Design review of the part built by this model. Coordinates are the model's own, in mm. Give positions to 0.01 mm unless a question says otherwise; leave off trailing zeros. Order: outer loops, then holes, each group sorted by start corner. A loop starts at its lowest first (then second) coordinate and runs counter-clockwise, first axis right, second up. Notation, with made-up numbers: M 49,-31 L 104,-31 A32 ccw 104,3 Z; hole C 33,75 d2. An arc over 180 degrees is marked long. Answer as a JSON object with one key per item and string values.
from build123d import *

# Parameters (mm, degrees)
PAD008_DEPTH          = 5
SKETCH022_W           = 88.2
SKETCH022_H           = 88.2
SKETCH022_R           = 2.5
PAD009_DEPTH          = 1.8
CHAMFER004_SIZE       = 1.2
PAD010_DEPTH          = 44.1
POCKET006_DEPTH       = 256.838707
POLARPATTERN002_COUNT = 8
CHAMFER005_SIZE       = 1.5
FILLET003_R           = 1.19


with BuildPart() as part:
    # Sketch021 → Pad008 (new body)
    with BuildSketch(Plane.XY.offset(-0.2)):
        Polygon((-42.9, 42.9), (-42.9, -42.9), (42.9, -42.9), (42.9, 42.9), (42.9, 44.1), (44.1, 44.1), (44.1, -44.1), (-44.1, -44.1), (-44.1, 44.1), (-42.9, 44.1), align=None)
    extrude(amount=-PAD008_DEPTH)

    # Sketch022 → Pad009 (join)
    with BuildSketch(Plane.XY.offset(-5.2)):
        Rectangle(SKETCH022_W, SKETCH022_H)
        with Locations((-35.7, 35.7)):
            Circle(SKETCH022_R, mode=Mode.SUBTRACT)
        with Locations((35.7, 35.7)):
            Circle(SKETCH022_R, mode=Mode.SUBTRACT)
        with Locations((35.7, -35.7)):
            Circle(SKETCH022_R, mode=Mode.SUBTRACT)
        with Locations((-35.7, -35.7)):
            Circle(SKETCH022_R, mode=Mode.SUBTRACT)
    extrude(amount=-PAD009_DEPTH)

    # Chamfer004
    chamfer004_edges = [part.edges().sort_by_distance(p)[0] for p in [
        (-38.2, 35.7, -7),
        (-38.2, -35.7, -7),
        (33.2, -35.7, -7),
        (33.2, 35.7, -7),
    ]]
    chamfer(chamfer004_edges, length=CHAMFER004_SIZE)

    # Sketch023 → Pad010 (join, symmetric)
    with BuildSketch(Plane.XZ):
        Polygon((42.9, -0.2), (42.9, -2.6), (41.7, -1.4), align=None)
        Polygon((-42.9, -0.2), (-42.9, -2.6), (-41.7, -1.4), align=None)
    extrude(amount=PAD010_DEPTH, both=True)

    # Sketch024 → Pocket006 (cut, through all)
    with BuildSketch(Plane.XY):
        with BuildLine():
            ThreePointArc((27.005677, 28.137047), (14.924654, 36.031302), (0.8, 38.991794))
            Line((0.8, 38.991794), (0.8, 27.785223))
            ThreePointArc((19.081434, 20.212805), (10.637351, 25.680837), (0.8, 27.785223))
            Line((19.081434, 20.212805), (27.005677, 28.137047))
        make_face()
        with BuildLine():
            ThreePointArc((17.950063, 19.081434), (10.025326, 24.203279), (0.8, 26.185223))
            Line((0.8, 14.978651), (0.8, 26.185223))
            ThreePointArc((10.025821, 11.157191), (5.740251, 13.858193), (0.8, 14.978651))
            Line((10.025821, 11.157191), (17.950063, 19.081434))
        make_face()
    pocket006 = extrude(amount=-POCKET006_DEPTH, mode=Mode.SUBTRACT)

    # PolarPattern002: Pocket006 ×8 about axis
    polarpattern002_axis = Axis((0, 0, 0), (0, 0, 1))
    for i in range(1, POLARPATTERN002_COUNT):
        add(pocket006.rotate(polarpattern002_axis, i * 360 / POLARPATTERN002_COUNT), mode=Mode.SUBTRACT)

    # Chamfer005
    chamfer005_edges = [part.edges().sort_by_distance(p)[0] for p in [
        (-44.1, 0, -7),
        (0, -44.1, -7),
        (44.1, 0, -7),
        (0, 44.1, -7),
    ]]
    chamfer(chamfer005_edges, length=CHAMFER005_SIZE)

    # Fillet003
    fillet003_edges = [part.edges().sort_by_distance(p)[0] for p in [
        (-44.1, 44.1, -2.85),
        (-44.1, -44.1, -2.85),
        (44.1, 44.1, -2.85),
        (44.1, -44.1, -2.85),
    ]]
    fillet(fillet003_edges, radius=FILLET003_R)


solid = part.part
(1) We need section C-C (x = -35.7). Write out the cut boundary in (y, z).
Checked values:
{"outline": "M -44.1,-5.5 L -42.6,-7 L -39.4,-7 L -38.2,-5.8 L -38.2,-5.2 L -42.9,-5.2 L -42.9,-0.2 L -44.1,-0.2 Z; M -33.2,-5.8 L -32,-7 L -15.7,-7 L -15.7,-5.2 L -33.2,-5.2 Z; M -0.8,-7 L 0.8,-7 L 0.8,-5.2 L -0.8,-5.2 Z; M 15.7,-7 L 32,-7 L 33.2,-5.8 L 33.2,-5.2 L 15.7,-5.2 Z; M 38.2,-5.8 L 39.4,-7 L 42.6,-7 L 44.1,-5.5 L 44.1,-5.2 L 38.2,-5.2 Z"}
(2) Draft analysis for pull direction X (two halves, no side actions). For faces 1 (the flat face through (-1, -44.1, -3)), 2 (the cylindrical face through (-5.81, -13.83, -6.09)), 3 (the cylindrical face through (33.2, 35.8, -5.5)), state which applies: +X half, -X half, draft (parallel to the pull), parting line (faces both ways), or undercut.
Checked values:
{"face 1": "draft", "face 2": "undercut", "face 3": "undercut"}
(3) We need section A-A (x = 12.5). Count the separate pieces of the cut face and the enclosed holes in it, plus the area to 3 significant figures.
Checked values:
{"separate pieces": "7", "enclosed holes": "0", "area": "74.0 mm^2"}
(4) To check wall thickness, follow L1, parallel to X at y = 23.5, z = -4.25; L2, parallel to X at y = -35.5, z = -5.75; L3, parallel to Y at x = -33.5, z = -6.5. State the ranges of each line that lie inside material, in increasing order. Write a range as from..to.
Checked values:
{"L1": "x = -44.1..-42.9, 42.9..44.1", "L2": "x = -43.85..-38.19, -33.21..-16.15, -0.8..0.8, 16.15..33.21, 38.19..43.85", "L3": "y = -43.1..-38.02, -33.38..-19.97, -0.8..0.8, 19.97..33.38, 38.02..43.1"}
(5) Insertion check: pin 1 (0.5 mm diameter, centred on y = 22, z = -6.5, fed in from +X); pin 2 (6.5 mm diameter, centred on x = 35.7, y = -35.7, fed in from -Z); pin 3 (1.4 mm diameter, centred on x = 35.5, z = -6.5, fed in from +Y); pin 4 (8 mm diameter, centred on x = -30.5, y = -15.5, fed in from -Z). Each pin has a flat end and moves straight along its axis. Give the tip position at first contact, or say it passes through.
Checked values:
{"pin 1": "stops at x = 43.35", "pin 2": "stops at z = -6.55", "pin 3": "stops at y = 43.8", "pin 4": "passes through"}
